Part model, mm, in its own coordinate system. Give positions to 0.01 mm unless a question says otherwise; leave off trailing zeros. Write each loop counter-clockwise with the first axis right and the second up, starting at its lowest first coordinate (ties: lowest second). Pieces come first, ordered by that corner, then holes.
from build123d import *

# Parameters (mm, degrees)
BRIDA_BASE4_DEPTH          = 1810
CORTAR_EXTRUIR1_DEPTH      = 1812.988923807
CORTAR_EXTRUIR1_DEPTH_BACK = 1812.988923807
DESDOBLAR1_DEPTH           = 1810
DESDOBLAR1_2_DEPTH         = 1810
CORTAR_EXTRUIR2_DEPTH      = 1813.989374608
CORTAR_EXTRUIR2_DEPTH_BACK = 1813.989374608


# Read off the part's stored shape, not the designer's step: Desdoblar1
# Sheet-metal steps are written as plain solids
with BuildPart() as part:
    # Croquis1 → Brida base4 (new body)
    with BuildSketch(Plane(origin=(0, 0, 0), x_dir=(1, 0, 0), z_dir=(0, 1, 0))):
        with BuildLine():
            Line((60.5, 0), (-57.8634, 0))
            ThreePointArc((-57.8634, 0), (-59.727757739, 0.772242261), (-60.5, 2.6366))
            Line((-60.5, 2.6366), (-60.5, 24.2634))
            ThreePointArc((-60.5, 24.2634), (-60.715745145, 24.784254855), (-61.2366, 25))
            Line((-61.2366, 25), (-80.5, 25))
            Line((-80.5, 25), (-80.5, 26.9))
            Line((-80.5, 26.9), (-61.2366, 26.9))
            ThreePointArc((-61.2366, 26.9), (-59.372242261, 26.127757739), (-58.6, 24.2634))
            Line((-58.6, 24.2634), (-58.6, 2.6366))
            ThreePointArc((-58.6, 2.6366), (-58.384254855, 2.115745145), (-57.8634, 1.9))
            Line((-57.8634, 1.9), (60.5, 1.9))
            Line((60.5, 1.9), (60.5, 0))
        make_face()
    extrude(amount=BRIDA_BASE4_DEPTH)

    # Croquis19 → Cortar-Extruir1 (cut, two sides: drawn at the far end of the back side and taken through both)
    with BuildSketch(Plane.XY.offset(-CORTAR_EXTRUIR1_DEPTH_BACK)):
        Polygon((60.5, 1000), (-39.5, 1810), (-39.5, 1900.089959651), (60.5, 1900.089959651), align=None)
    extrude(amount=CORTAR_EXTRUIR1_DEPTH + CORTAR_EXTRUIR1_DEPTH_BACK, mode=Mode.SUBTRACT)

    # Desdoblar1 outline → Desdoblar1 (cut)
    with BuildSketch(Plane(origin=(0, 0, 0), x_dir=(1, 0, 0), z_dir=(0, 1, 0))):
        with BuildLine():
            ThreePointArc((-60.5, 2.6366), (-60.473622072, 2.264578098), (-60.395016084, 1.9))
            Line((-60.395016084, 1.9), (-57.8634, 1.9))
            ThreePointArc((-57.8634, 1.9), (-58.384254855, 2.115745145), (-58.6, 2.6366))
            Line((-58.6, 2.6366), (-58.6, 24.2634))
            ThreePointArc((-58.6, 24.2634), (-59.372242261, 26.127757739), (-61.2366, 26.9))
            Line((-61.2366, 26.9), (-80.5, 26.9))
            Line((-80.5, 26.9), (-80.5, 25))
            Line((-80.5, 25), (-61.2366, 25))
            ThreePointArc((-61.2366, 25), (-60.715745145, 24.784254855), (-60.5, 24.2634))
            Line((-60.5, 24.2634), (-60.5, 2.6366))
        make_face()
    extrude(amount=DESDOBLAR1_DEPTH, mode=Mode.SUBTRACT)

    # Desdoblar1 2 outline → Desdoblar1 2 (add)
    with BuildSketch(Plane(origin=(0, 0, 0), x_dir=(1, 0, 0), z_dir=(0, 1, 0))):
        with BuildLine():
            Line((-104.05221017, 0), (-57.8634, 0))
            ThreePointArc((-57.8634, 0), (-59.446046517, 0.527835063), (-60.395016084, 1.9))
            Line((-60.395016084, 1.9), (-104.05221017, 1.9))
            Line((-104.05221017, 1.9), (-104.05221017, 0))
        make_face()
    extrude(amount=DESDOBLAR1_2_DEPTH)

    # Croquis20 → Cortar-Extruir2 (cut, two sides: drawn at the far end of the back side and taken through both)
    with BuildSketch(Plane.XY.offset(-CORTAR_EXTRUIR2_DEPTH_BACK)):
        with BuildLine():
            ThreePointArc((-82.464157627, 1805.95), (-82.742406185, 1805.278248558), (-83.414157627, 1805))
            Line((-83.414157627, 1805), (-83.514157627, 1805))
            ThreePointArc((-83.514157627, 1805), (-84.185909069, 1805.278248558), (-84.464157627, 1805.95))
            Line((-84.464157627, 1805.95), (-84.464157627, 1810))
            Line((-84.464157627, 1810), (-82.464157627, 1810))
            Line((-82.464157627, 1810), (-82.464157627, 1805.95))
        make_face()
        with BuildLine():
            ThreePointArc((-58.188052542, 1805.95), (-58.4663011, 1805.278248558), (-59.138052542, 1805))
            Line((-59.138052542, 1805), (-59.238052542, 1805))
            ThreePointArc((-59.238052542, 1805), (-59.909803985, 1805.278248558), (-60.188052542, 1805.95))
            Line((-60.188052542, 1805.95), (-60.188052542, 1810))
            Line((-60.188052542, 1810), (-58.188052542, 1810))
            Line((-58.188052542, 1810), (-58.188052542, 1805.95))
        make_face()
        with BuildLine():
            ThreePointArc((-84.464157627, 4.05), (-84.185909069, 4.721751442), (-83.514157627, 5))
            Line((-83.514157627, 5), (-83.414157627, 5))
            ThreePointArc((-83.414157627, 5), (-82.742406185, 4.721751442), (-82.464157627, 4.05))
            Line((-82.464157627, 4.05), (-82.464157627, 0))
            Line((-82.464157627, 0), (-84.464157627, 0))
            Line((-84.464157627, 0), (-84.464157627, 4.05))
        make_face()
        with BuildLine():
            ThreePointArc((-60.188052542, 4.05), (-59.909803985, 4.721751442), (-59.238052542, 5))
            Line((-59.238052542, 5), (-59.138052542, 5))
            ThreePointArc((-59.138052542, 5), (-58.4663011, 4.721751442), (-58.188052542, 4.05))
            Line((-58.188052542, 4.05), (-58.188052542, 0))
            Line((-58.188052542, 0), (-60.188052542, 0))
            Line((-60.188052542, 0), (-60.188052542, 4.05))
        make_face()
    extrude(amount=CORTAR_EXTRUIR2_DEPTH + CORTAR_EXTRUIR2_DEPTH_BACK, mode=Mode.SUBTRACT)


solid = part.part
1) Flat gauge pins, fed straight in: P1, Ø0.6, axis at y = 1808.5, z = -1.5, coming from the +X side; P2, Ø1, axis at y = 1807.5, z = -1, coming from the +X side. Where does each tip first touch, or does it go through?
Check result:
P1: stops at x = -39.28
P2: stops at x = -39.13
2) Saw through at C-C (y = 1321.5). Write the cut outline in (x, z), and give its area (3 significant figures).
Check result:
outline: (-104.05, -1.9) - (20.81, -1.9) - (20.81, 0) - (-104.05, 0) - close
area: 237 mm2
3) Drill centre lines: L1, parallel to Y at x = -83, z = -1.8; L2, parallel to Y at x = -59.5, z = -1.1; L3, parallel to X at y = 1042.5, z = -1.5. Where is each one in solid material? Low to high.
Check result:
L1: y = 4.9 to 1805.1
L2: y = 4.96 to 1805.04
L3: x = -104.05 to 55.25
4) Saw through at B-B (x = 39.5). Write the cut outline in (y, z).
Check result:
outline: (0, -1.9) - (1170.1, -1.9) - (1170.1, 0) - (0, 0) - close
